Autodesk Inventor part; units mm, degrees
ref_plane "YZ Plane" through (0, 0, 0) normal (1, 0, 0) x (0, 1, 0)
ref_plane "XZ Plane" through (0, 0, 0) normal (0, 1, 0) x (-1, 0, 0)
ref_plane "XY Plane" through (0, 0, 0) normal (0, 0, 1) x (1, 0, 0)
sketch "Sketch1" plane through (0, 0, 0) normal (0, 1, 0) x (-1, 0, 0)
  line L0 (-20, 20) -> (20, 20)
  line L1 (20, 20) -> (20, -20)
  line L2 (20, -20) -> (-20, -20)
  line L3 (-20, -20) -> (-20, 20)
  line L4 (-20, 20) -> (20, -20) construction
  line L5 (20, 20) -> (-20, -20) construction
  circle A0 centre (15, -15) radius 1.5
  circle A1 centre (-15, -15) radius 1.5
  circle A2 centre (-15, 15) radius 1.5
  circle A3 centre (15, 15) radius 1.5
  line L6 (15, 15) -> (15, -15) construction
  line L7 (-15, -15) -> (15, -15) construction
  line L8 (-15, -15) -> (-15, 15) construction
  line L9 (-20, 20) -> (-49, 20)
  line L10 (-49, 20) -> (-49, -20)
  line L11 (-49, -20) -> (-20, -20)
  circle A4 centre (0, 0) radius 3.5
  line L12 (20, 20) -> (20, 25)
  line L13 (20, 25) -> (-49, 25)
  line L14 (-49, 25) -> (-49, 20)
  line L15 (-34.5, -20) -> (-34.5, -10) construction
  line L16 (-34.5, -10) -> (-34.5, 10) construction
  circle A5 centre (-34.5, -10) radius 1.6
  circle A6 centre (-34.5, 10) radius 1.6
  dimension "d0" = 40
  dimension "d1" = 40
  dimension "d2" = 30
  dimension "d3" = 3
  dimension "d26" = 7
  dimension "d27" = 29
  dimension "d29" = 5
  dimension "d40" = 10
  dimension "d41" = 20
  dimension "d42" = 3.2
sketch "Sketch1 outline for Extrusion1" plane through (0, 0, 0) normal (0, 1, 0) x (-1, 0, 0)
  line L0 (-49, 25) -> (-49, -20)
  line L1 (-49, -20) -> (20, -20)
  line L2 (20, -20) -> (20, 25)
  line L3 (20, 25) -> (-49, 25)
  circle A0 centre (15, 15) radius 1.5
  circle A1 centre (0, 0) radius 3.5
  circle A2 centre (-34.5, -10) radius 1.6
  circle A3 centre (-15, -15) radius 1.5
  circle A4 centre (15, -15) radius 1.5
  circle A5 centre (-34.5, 10) radius 1.6
  circle A6 centre (-15, 15) radius 1.5
extrude "Extrusion1" add sketch "Sketch1 outline for Extrusion1" along normal blind 5
sketch "Sketch1 outline for Extrusion4" plane through (0, 0, 0) normal (0, 1, 0) x (-1, 0, 0)
  line L0 (-49, 25) -> (-49, 20)
  line L1 (20, 25) -> (-49, 25)
  line L2 (20, 20) -> (20, 25)
  line L3 (-20, 20) -> (20, 20)
  line L4 (-49, 20) -> (-20, 20)
extrude "Extrusion4" add sketch "Sketch1 outline for Extrusion4" against normal blind 42
sketch "Sketch2" plane through (-20, 5, 25) normal (0, 0, 1) x (1, 0, 0)
  line L0 (69, -47) -> (69, 0)
  line L1 (0, 0) -> (69, 0)
  line L2 (0, -47) -> (0, 0)
  line L3 (69, -47) -> (0, -47)
  line L4 (69, -47) -> (40, -47)
  line L5 (40, -47) -> (40, 0)
  line L6 (40, 0) -> (69, 0)
  line L7 (69, 0) -> (69, -47)
  circle A0 centre (54.5, -26) radius 11.5
  line L8 (54.5, -26) -> (54.5, -47) construction
  line L9 (69, -47) -> (0, -47)
  line L10 (43, -32.639528) -> (43, -19.360472)
  line L11 (43, -19.360472) -> (54.5, -12.720944)
  line L12 (54.5, -12.720944) -> (66, -19.360472)
  line L13 (66, -19.360472) -> (66, -32.639528)
  line L14 (66, -32.639528) -> (54.5, -39.279056)
  line L15 (54.5, -39.279056) -> (43, -32.639528)
  line L16 (54.5, -39) -> (62, -39) construction
  line L17 (54.5, -39) -> (47, -39) construction
  circle A1 centre (62, -39) radius 1.6
  circle A2 centre (47, -39) radius 1.6
  point P0 (20, -5)
  point P1 (54.5, -26)
  point P2 (48.75, -35.959292)
  point P3 (60.25, -35.959292)
  point P4 (43, -26)
  point P5 (66, -26)
  point P6 (60.25, -16.040708)
  point P7 (48.75, -16.040708)
  dimension "d32" = 29
  dimension "d33" = 21
  dimension "d34" = 23
  dimension "d37" = 3.2
  dimension "d39" = 8
  dimension "d46" = 15
sketch "Sketch2 outline for Extrusion5" plane through (-20, 5, 25) normal (0, 0, 1) x (1, 0, 0)
  circle A0 centre (62, -39) radius 1.6
  circle A1 centre (47, -39) radius 1.6
  circle A2 centre (54.5, -26) radius 11.5
extrude "Extrusion5" cut sketch "Sketch2 outline for Extrusion5" against normal up to surface (5 mm away)
chamfer "Chamfer4" distance 40 angle 45 1 edges at (-20, -42, 22.5)
chamfer "Chamfer5" distance 2 distance2 5 1 edges at (23, -21, 25)
sketch "Sketch3" plane through (0, 5, 0) normal (0, 1, 0) x (1, 0, 0)
  point P0 (0, 0)
properties part number "Tensioner Top_3DPrint"
Work out the finished part from the listing and answer in its coordinate system (mm). A direction names the side the tool comes from. Give positions to 0.01 mm unless a question says otherwise; leave off trailing zeros. Loops run counter-clockwise (first coordinate to the right, second up) from the corner with the lowest first, then second, coordinate; pieces in that order, holes last. Notation, with made-up numbers: (17.25, -6.5) -> (54.25, -6.5) arc R18 ccw to (54.25, 0.5) -> close; hole circle Ø11 at (73, 76). An arc over 180 degrees is marked (long way). Use a Markdown table: item, result. Add a question column.
1) The part is cut by section C-C, the plane x = 0. Determine the outline of the cut face in (y, z).
2) The part is cut by section D-D, the plane y = -21. Determine the outline of the cut face in (x, z), plus the area to 3 significant figures.
3) For a pull along Y with two mould halves and no side action, classify faces 3 (the flat face through (0, -22, 23)), 4 (the cylindrical face through (26.65, -35.56, 22.54)), 5 (the cylindrical face through (-13.5, 2.46, 14.93)) as +Y half, -Y half, draft (parallel to the pull), parting line (faces both ways), or undercut.
4) Which of the six approach directions +Z, -Z, +X, -X, +Y, -Y give full straight-line access (tool end or side, diameter ignored) to faces 1 (the flat face through (15, 0, 0)), 2 (the flat face through (-20, 2, 2))?
5) The part is cut by section A-A, the plane x = 34.5. Determine the outline of the cut face in (y, z).
6) Consider line 1 along Z through (x, y) = (34.5, 2.45); line 2 along Z through (x, y) = (-15, 3.55); line 3 along X through (y, z) = (-34, 22.35). Determine where each line is inside the solid, lowest interval first.
7) Each of these flat-tipped pins is pushed along its axis until it touches: P1, Ø3, axis at x = 2.5, z = -11.5, coming from the -Y side; P2, Ø5, axis at x = 27, y = -34, coming from the -Z side. Where does it stop, or does it pass through?
8) The part is cut by section B-B, the plane z = -10. Determine the outline of the cut face in (x, y).
Reported:
| question | item | result |
|---|---|---|
| 1 | outline | (-22, 20) -> (0, 20) -> (0, 3.5) -> (5, 3.5) -> (5, 25) -> (-22, 25) -> close; (0, -20) -> (5, -20) -> (5, -3.5) -> (0, -3.5) -> close |
| 2 | outline | (-1, 20) -> (23, 20) -> (21, 25) -> (-1, 25) -> close; (46, 20) -> (49, 20) -> (49, 25) -> (48, 25) -> close |
| 2 | area | 125 mm^2 |
| 3 | face 3 | -Y half |
| 3 | face 4 | undercut |
| 3 | face 5 | draft |
| 4 | face 1 | -Z, +X, -X, -Y |
| 4 | face 2 | +Z, -Z, -X, +Y, -Y |
| 5 | outline | (-42, 20) -> (-32.5, 20) -> (-34.5, 25) -> (-42, 25) -> close; (-9.5, 20) -> (0, 20) -> (0, 11.6) -> (5, 11.6) -> (5, 25) -> (-7.5, 25) -> close; (0, -20) -> (5, -20) -> (5, -11.6) -> (0, -11.6) -> close; (0, -8.4) -> (5, -8.4) -> (5, 8.4) -> (0, 8.4) -> close |
| 6 | line 1 | z = -20 to -11.6, -8.4 to 8.4, 11.6 to 25 |
| 6 | line 2 | z = -20 to -16.5, -13.5 to 13.5, 16.5 to 25 |
| 6 | line 3 | x = 12 to 25.4, 28.6 to 40.4, 43.6 to 49 |
| 7 | P1 | stops at y = 0 |
| 7 | P2 | stops at z = 20 |
| 8 | outline | (-20, 0) -> (32.9, 0) -> (32.9, 5) -> (-20, 5) -> close; (36.1, 0) -> (49, 0) -> (49, 5) -> (36.1, 5) -> close |
